The model under review builds one solid part; all positions refer to its coordinate system, in mm. A direction names the side the tool comes from. Round coordinates to 2 decimals unless told otherwise and drop trailing zeros. Order: outer loops, then holes, each group sorted by start corner. A loop starts at its lowest first (then second) coordinate and runs counter-clockwise, first axis right, second up. Notation, with made-up numbers: (56.5, 67) -> (91.5, 67) arc R19 cw to (91.5, 83) -> close; hole circle Ø1 at (45.5, 48). An arc over 180 degrees is marked (long way). Use a Markdown table: item, result. Add a question column.
Autodesk Fusion 360 part; units mm, degrees
sketch "Sketch1" plane through (0, 0, 0) normal (0, 0, 1) x (1, 0, 0)
  line L0 (0, 0) -> (50, 0)
  line L1 (50, 0) -> (50, 27)
  line L2 (50, 27) -> (0, 27)
  line L3 (0, 27) -> (0, 0)
  dimension "d1" = 27
  dimension "d2" = 50
extrude "Extrude1" add sketch "Sketch1" against normal blind 5
extrude "Extrude2" cut 1 faces at (16.6667, 18, -5) along direction (0, 0, 1) blind 3
sketch "Sketch3" plane through (0, 0, 0) normal (0, 0, 1) x (1, 0, 0)
  line L0 (0, 27) -> (0, 0)
  line L1 (0, 0) -> (50, 0)
  line L2 (50, 0) -> (50, 27)
  line L3 (50, 27) -> (0, 27)
  line L4 (10, 24) -> (40, 24)
  line L5 (40, 24) -> (40, 3)
  line L6 (40, 3) -> (10, 3)
  line L7 (10, 3) -> (10, 24)
  line L8 (36, 5) -> (14, 5)
  line L9 (12, 7) -> (12, 20)
  line L10 (14, 22) -> (36, 22)
  line L11 (38, 20) -> (38, 7)
  arc A0 (38, 20) -> (36, 22) centre (36, 20) ccw
  arc A1 (36, 5) -> (38, 7) centre (36, 7) ccw
  arc A2 (12, 7) -> (14, 5) centre (14, 7) ccw
  arc A3 (14, 22) -> (12, 20) centre (14, 20) ccw
  dimension "d10" = 21
  dimension "d11" = 3
  dimension "d12" = 30
  dimension "d13" = 10
  dimension "d22" = 2
extrude "Extrude3" add 1 faces at (16.6667, 18, -2) along direction (0, 0, -1) blind 1
extrude "Extrude4" cut sketch "Sketch3" against normal blind 2 contours L8 L9 L10 L11 A0 A1 A2 A3
sketch "Sketch5" plane through (0, 0, 0) normal (0, 0, 1) x (1, 0, 0)
  line L0 (14, 22) -> (36, 22)
  arc A0 (38, 20) -> (36, 22) centre (36, 20) ccw
  line L1 (38, 20) -> (38, 7)
  arc A1 (36, 5) -> (38, 7) centre (36, 7) ccw
  line L2 (36, 5) -> (14, 5)
  arc A2 (12, 7) -> (14, 5) centre (14, 7) ccw
  line L3 (12, 7) -> (12, 20)
  arc A3 (14, 22) -> (12, 20) centre (14, 20) ccw
  line L4 (0, 27) -> (0, 0)
  line L5 (0, 0) -> (50, 0)
  line L6 (50, 0) -> (50, 27)
  line L7 (50, 27) -> (0, 27)
  line L8 (14, 24) -> (36, 24)
  arc A4 (40, 20) -> (36, 24) centre (36, 20) ccw
  line L9 (40, 20) -> (40, 7)
  arc A5 (36, 3) -> (40, 7) centre (36, 7) ccw
  line L10 (36, 3) -> (14, 3)
  arc A6 (10, 7) -> (14, 3) centre (14, 7) ccw
  line L11 (10, 7) -> (10, 20)
  arc A7 (14, 24) -> (10, 20) centre (14, 20) ccw
  dimension "d23" = 2
extrude "Extrude5" cut sketch "Sketch5" against normal blind 1 contours L8 A4 L9 A5 L10 A6 L11 A7
sketch "Sketch6" plane through (0, 0, -2) normal (0, 0, 1) x (1, 0, 0)
  arc A0 (38, 20) -> (36, 22) centre (36, 20) ccw
  line L0 (36, 22) -> (14, 22)
  arc A1 (14, 22) -> (12, 20) centre (14, 20) ccw
  line L1 (12, 20) -> (12, 7)
  arc A2 (12, 7) -> (14, 5) centre (14, 7) ccw
  line L2 (14, 5) -> (36, 5)
  arc A3 (36, 5) -> (38, 7) centre (36, 7) ccw
  line L3 (38, 7) -> (38, 20)
  line L4 (18, 18) -> (32, 18)
  line L5 (32, 18) -> (32, 9)
  line L6 (32, 9) -> (18, 9)
  line L7 (18, 9) -> (18, 18)
  dimension "d28" = 4
  dimension "d29" = 4
  dimension "d30" = 9
  dimension "d31" = 6
  dimension "d32" = 6
extrude "Extrude6" cut sketch "Sketch6" against normal blind 10 contours L4 L5 L6 L7
sketch "Sketch7" plane through (0, 0, 0) normal (0, 0, 1) x (1, 0, 0)
  line L0 (14, 24) -> (36, 24)
  arc A0 (40, 20) -> (36, 24) centre (36, 20) ccw
  line L1 (40, 20) -> (40, 7)
  arc A1 (36, 3) -> (40, 7) centre (36, 7) ccw
  line L2 (36, 3) -> (14, 3)
  arc A2 (10, 7) -> (14, 3) centre (14, 7) ccw
  line L3 (10, 7) -> (10, 20)
  arc A3 (14, 24) -> (10, 20) centre (14, 20) ccw
  line L4 (0, 27) -> (0, 0)
  line L5 (0, 0) -> (50, 0)
  line L6 (50, 0) -> (50, 27)
  line L7 (50, 27) -> (0, 27)
  line L8 (0, 27) -> (5, 27)
  line L9 (5, 27) -> (5, 0)
  line L10 (5, 13.5) -> (0, 13.5)
  line L11 (2.5, 13.5) -> (2.5, 27)
  line L12 (2.5, 13.5) -> (2.5, 20.25)
  circle A4 centre (2.5, 20.25) radius 1.5
  line L13 (2.5, 13.5) -> (2.5, 6.75)
  circle A5 centre (2.5, 6.75) radius 1.5
  line L14 (50, 27) -> (45, 27)
  line L15 (45, 27) -> (45, 0)
  line L16 (45, 0) -> (50, 0)
  line L17 (50, 0) -> (50, 27)
  line L18 (45, 13.5) -> (50, 13.5)
  line L19 (47.5, 13.5) -> (47.5, 20.25)
  circle A6 centre (47.5, 20.25) radius 1.5
  line L20 (47.5, 13.5) -> (47.5, 6.75)
  circle A7 centre (47.5, 6.75) radius 1.5
  dimension "d35" = 3
  dimension "d36" = 6.75
  dimension "d37" = 3
  dimension "d40" = 6.75
  dimension "d41" = 3
  dimension "d42" = 6.75
  dimension "d43" = 3
extrude "Extrude7" cut sketch "Sketch7" against normal blind 10 contours A5 | L11 L12 A4 | L11 L12 A4
extrude "Extrude8" cut sketch "Sketch7" against normal blind 11 contours A5 | L11 L12 A4 | L11 L12 A4 | A6 | A7
extrude "Extrude9" add 1 faces at (36, 15, -2) along direction (0, 0, 1) blind 2
extrude "Extrude10" cut 1 faces at (22.6667, 24, -3) along direction (0, 0, 1) blind 1
extrude "Extrude11" add 1 faces at (33.3333, 27, -0.6667) along direction (0, 1, 0) blind 2
extrude "Extrude12" add 1 faces at (16.6667, 0, -0.6667) along direction (0, -1, 0) blind 1
Q1. Add section A-A (z = -0.45). Write out the cut boundary in (x, y), then the cut area to 3 significant figures.
Q2. Machinability: for faces 1 (the flat face through (18, 13, -1)), 2 (the cylindrical face through (11.203, 22.859, -0.493)), 3 (the flat face through (25, 21, -2)), which of the approach directions +Z, -Z, +X, -X, +Y, -Y give a long, thin tool a straight path to every point of the face, cutting with its end or side? Answer none if there is none.
Q3. Wall thickness on line 1 (X direction, y = 20.25, z = -1.3); line 2 (X direction, y = 17, z = -0.2); line 3 (Y direction, x = 2.5, z = -0.95): over which ranges is each line inside the solid? List them lowest first. Write a range as [from, to].
Q4. Add section B-B (x = 47.5). Write out the cut boundary in (y, z), then the cut area to 3 significant figures.
Q5. Mouldability with a two-part tool opening along X and no side actions: class faces 4 (the flat face through (24.7, 24.2, 0)), 5 (the flat face through (50, 14, -1)), 6 (the flat face through (32, 14, -1)), 7 (the cylindrical face through (12.57, 21.4, -0.51)) as pulls with the +X half, pulls with the -X half, needs draft (parallel to the pull), parting line crosses it, or undercut.
Q6. Add section D-D (x = 11). Write out the cut boundary in (y, z).
Q7. Add section C-C (y = 16). Write out the cut boundary in (x, z), then the cut area to 3 significant figures.
Report:
| question | item | result |
|---|---|---|
| 1 | outline | (0, -1) -> (50, -1) -> (50, 29) -> (0, 29) -> close; (12, 7) arc R2 ccw to (14, 5) -> (36, 5) arc R2 ccw to (38, 7) -> (38, 20) arc R2 ccw to (36, 22) -> (14, 22) arc R2 ccw to (12, 20) -> close; hole circle Ø3 at (2.5, 6.75); hole circle Ø3 at (2.5, 20.25); hole (10, 7) arc R4 ccw to (14, 3) -> (36, 3) arc R4 ccw to (40, 7) -> (40, 20) arc R4 ccw to (36, 24) -> (14, 24) arc R4 ccw to (10, 20) -> close; hole (18, 9) -> (32, 9) -> (32, 18) -> (18, 18) -> close; hole circle Ø3 at (47.5, 6.75); hole circle Ø3 at (47.5, 20.25) |
| 1 | area | 1,170 mm² |
| 2 | face 1 | +Z, -Z |
| 2 | face 2 | +Z |
| 2 | face 3 | -Z, +X, -X, +Y, -Y |
| 3 | line 1 | x = [0, 1], [4, 46], [49, 50] |
| 3 | line 2 | x = [0, 10], [12, 18], [32, 38], [40, 50] |
| 3 | line 3 | y = [-1, 5.25], [8.25, 18.75], [21.75, 29] |
| 4 | outline | (-1, -2) -> (5.25, -2) -> (5.25, 0) -> (-1, 0) -> close; (8.25, -2) -> (18.75, -2) -> (18.75, 0) -> (8.25, 0) -> close; (21.75, -2) -> (29, -2) -> (29, 0) -> (21.75, 0) -> close |
| 4 | area | 48.0 mm² |
| 5 | face 4 | needs draft |
| 5 | face 5 | pulls with the +X half |
| 5 | face 6 | undercut |
| 5 | face 7 | undercut |
| 6 | outline | (-1, -2) -> (29, -2) -> (29, 0) -> (22.65, 0) -> (22.65, -1) -> (4.35, -1) -> (4.35, 0) -> (-1, 0) -> close |
| 7 | outline | (0, -2) -> (18, -2) -> (18, 0) -> (12, 0) -> (12, -1) -> (10, -1) -> (10, 0) -> (0, 0) -> close; (32, -2) -> (50, -2) -> (50, 0) -> (40, 0) -> (40, -1) -> (38, -1) -> (38, 0) -> (32, 0) -> close |
| 7 | area | 68.0 mm² |
